Here's how the part is built. I have some questions about the finished solid (model axes, mm). Face numbers are marked on the shaded views. Give positions to 0.01 mm unless a question says otherwise; leave off trailing zeros. Put each result on its own line as item: value. Start each with the question number.
from build123d import *

# Parameters (mm, degrees)
SKETCH1_R           = 50
SKETCH1_R_2         = 1
BOSS_EXTRUDE1_DEPTH = 20


with BuildPart() as part:
    # Sketch1 → Boss-Extrude1 (new body)
    with BuildSketch(Plane.XY):
        Circle(SKETCH1_R)
        Circle(SKETCH1_R_2, mode=Mode.SUBTRACT)
    extrude(amount=BOSS_EXTRUDE1_DEPTH)

    # Sketch2 → Cut-Revolve1 (revolve, cut)
    with BuildSketch(Plane(origin=(0, 0, 0), x_dir=(0, 0, -1), z_dir=(1, 0, 0)), mode=Mode.PRIVATE) as cut_revolve1_sk:
        Polygon((-18, 50), (-17, 49), (-12, 49), (-11, 50), align=None)
        Polygon((-9, 50), (-8, 49), (-3, 49), (-2, 50), align=None)
    revolve(cut_revolve1_sk.sketch.rotate(Axis((0, 0, 1011.858451466), (0, 0, -1)), 90), axis=Axis((0, 0, 1011.858451466), (0, 0, -1)), mode=Mode.SUBTRACT)

    # Sketch4 → Cut-Revolve2 (revolve, cut)
    with BuildSketch(Plane(origin=(0, 0, 0), x_dir=(0, 0, -1), z_dir=(1, 0, 0)), mode=Mode.PRIVATE) as cut_revolve2_sk:
        with BuildLine():
            Line((-3, 0), (-3, 25))
            ThreePointArc((-3, 25), (-7.97918472, 37.02081528), (-20, 42))
            Line((-20, 42), (-20, 0))
            Line((-20, 0), (-3, 0))
        make_face()
    revolve(cut_revolve2_sk.sketch.rotate(Axis((0, 0, 1012), (0, 0, -1)), 90), axis=Axis((0, 0, 1012), (0, 0, -1)), mode=Mode.SUBTRACT)


solid = part.part
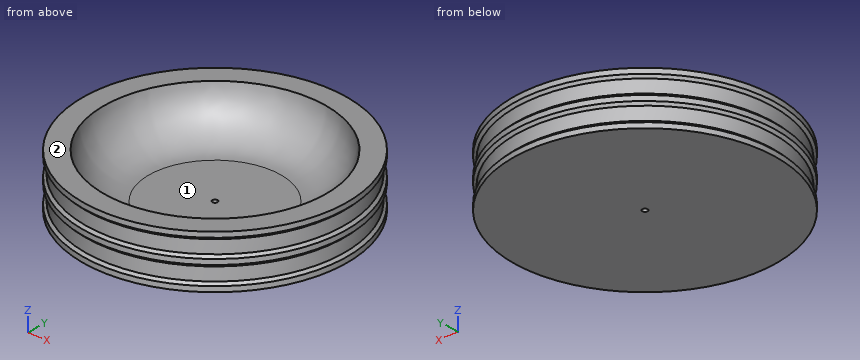
1) I need wall thicknesses on line 1 (X direction, y = 0, z = 1.15); line 2 (Z direction, x = 42.5, y = -26); line 3 (Z direction, x = -6, y = -10.5). Which ranges of each line are inside material? Lowest first, please.
2) I'm going to push flat-ended pins straight in: P1, Ø1, axis at y = 8.5, z = 15.5, coming from the -X side; P2, Ø1.5, axis at y = -21.5, z = 13, coming from the -X side; P3, Ø6, axis at y = 31.5, z = 8, coming from the +X side. Where does each tip first touch, or does it pass through?
3) Thinking about a two-plate mould opening in X: for the marked faces 1 and 2, which applies, pulls with the +X half, pulls with the -X half, needs draft (parallel to the pull), parting line crosses it, or undercut?
Ans:
1. line 1: x = -50 to -1, 1 to 50
1. line 2: z = 0 to 2.18, 8.82 to 11.18, 17.82 to 20
1. line 3: z = 0 to 3
2. P1: stops at x = -48.34
2. P2: stops at x = -44.39
2. P3: stops at x = 40.96
3. face 1: undercut
3. face 2: needs draft
